Build history of the part. All positions in model axes, mm. A direction names the side the tool comes from. Give positions to 0.01 mm unless a question says otherwise; leave off trailing zeros. Order: outer loops, then holes, each group sorted by start corner. A loop starts at its lowest first (then second) coordinate and runs counter-clockwise, first axis right, second up. Notation, with made-up numbers: (70.5, -30.5) - (101.5, -30.5) arc R24 cw to (101.5, 8.5) - close; hole circle Ø6 at (-9, 7). An arc over 180 degrees is marked (long way). Use a Markdown table: item, result.
from build123d import *

# Parameters (mm, degrees)
SKETCH1_R           = 6.1
BOSS_EXTRUDE1_DEPTH = 4
BOSS_EXTRUDE2_START = 4
SKETCH1_3_R         = 20
SKETCH1_3_R_2       = 16
BOSS_EXTRUDE2_DEPTH = 12
BOSS_EXTRUDE3_DEPTH = 2
SKETCH1_5_R         = 2
BOSS_EXTRUDE4_DEPTH = 6
BOSS_EXTRUDE5_START = 4
SKETCH1_6_R         = 1.5
BOSS_EXTRUDE5_DEPTH = 10


with BuildPart() as part:
    # Sketch1 → Boss-Extrude1 (new body)
    with BuildSketch(Plane(origin=(0, 0, 0), x_dir=(1, 0, 0), z_dir=(0, 1, 0))):
        with BuildLine():
            Line((-24, 20), (-28, 20))
            Line((-28, 20), (-28, -20))
            Line((-28, -20), (-24, -20))
            ThreePointArc((-24, -20), (-21.171572875, -21.171572875), (-20, -24))
            Line((-20, -24), (-20, -28))
            Line((-20, -28), (20, -28))
            Line((20, -28), (20, -24))
            ThreePointArc((20, -24), (21.171572875, -21.171572875), (24, -20))
            Line((24, -20), (28, -20))
            Line((28, -20), (28, 20))
            Line((28, 20), (24, 20))
            ThreePointArc((24, 20), (21.171572875, 21.171572875), (20, 24))
            Line((20, 24), (20, 28))
            Line((20, 28), (-20, 28))
            Line((-20, 28), (-20, 24))
            ThreePointArc((-20, 24), (-21.171572875, 21.171572875), (-24, 20))
        make_face()
        Circle(SKETCH1_R, mode=Mode.SUBTRACT)
    extrude(amount=BOSS_EXTRUDE1_DEPTH)

    # Sketch1_3 → Boss-Extrude2 (add)
    with BuildSketch(Plane(origin=(0, 0, 0), x_dir=(1, 0, 0), z_dir=(0, 1, 0)).offset(BOSS_EXTRUDE2_START)):
        Circle(SKETCH1_3_R)
        Circle(SKETCH1_3_R_2, mode=Mode.SUBTRACT)
    extrude(amount=BOSS_EXTRUDE2_DEPTH)

    # Sketch1_4 → Boss-Extrude3 (add)
    with BuildSketch(Plane(origin=(0, 0, 0), x_dir=(1, 0, 0), z_dir=(0, 1, 0))):
        with BuildLine():
            Line((24, 30), (-24, 30))
            ThreePointArc((-24, 30), (-28.242640687, 28.242640687), (-30, 24))
            Line((-30, 24), (-30, -24))
            ThreePointArc((-30, -24), (-28.242640687, -28.242640687), (-24, -30))
            Line((-24, -30), (24, -30))
            ThreePointArc((24, -30), (28.242640687, -28.242640687), (30, -24))
            Line((30, -24), (30, 24))
            ThreePointArc((30, 24), (28.242640687, 28.242640687), (24, 30))
        make_face()
        with BuildLine():
            Line((-28, 20), (-28, 24))
            ThreePointArc((-28, 24), (-26.828427125, 26.828427125), (-24, 28))
            Line((-24, 28), (-20, 28))
            Line((-20, 28), (20, 28))
            Line((20, 28), (24, 28))
            ThreePointArc((24, 28), (26.828427125, 26.828427125), (28, 24))
            Line((28, 24), (28, 20))
            Line((28, 20), (28, -20))
            Line((28, -20), (28, -24))
            ThreePointArc((28, -24), (26.828427125, -26.828427125), (24, -28))
            Line((24, -28), (20, -28))
            Line((20, -28), (-20, -28))
            Line((-20, -28), (-24, -28))
            ThreePointArc((-24, -28), (-26.828427125, -26.828427125), (-28, -24))
            Line((-28, -24), (-28, -20))
            Line((-28, -20), (-28, 20))
        make_face(mode=Mode.SUBTRACT)
    extrude(amount=BOSS_EXTRUDE3_DEPTH)

    # Sketch1_5 → Boss-Extrude4 (add)
    with BuildSketch(Plane(origin=(0, 0, 0), x_dir=(1, 0, 0), z_dir=(0, 1, 0))):
        with BuildLine():
            Line((-24, -20), (-28, -20))
            Line((-28, -20), (-28, -24))
            ThreePointArc((-28, -24), (-26.828427125, -26.828427125), (-24, -28))
            Line((-24, -28), (-20, -28))
            Line((-20, -28), (-20, -24))
            ThreePointArc((-20, -24), (-21.171572875, -21.171572875), (-24, -20))
        make_face()
        with Locations((-24, -24)):
            Circle(SKETCH1_5_R, mode=Mode.SUBTRACT)
        with BuildLine():
            Line((20, -24), (20, -28))
            Line((20, -28), (24, -28))
            ThreePointArc((24, -28), (26.828427125, -26.828427125), (28, -24))
            Line((28, -24), (28, -20))
            Line((28, -20), (24, -20))
            ThreePointArc((24, -20), (21.171572875, -21.171572875), (20, -24))
        make_face()
        with Locations((24, -24)):
            Circle(SKETCH1_5_R, mode=Mode.SUBTRACT)
        with BuildLine():
            Line((24, 28), (20, 28))
            Line((20, 28), (20, 24))
            ThreePointArc((20, 24), (21.171572875, 21.171572875), (24, 20))
            Line((24, 20), (28, 20))
            Line((28, 20), (28, 24))
            ThreePointArc((28, 24), (26.828427125, 26.828427125), (24, 28))
        make_face()
        with Locations((24, 24)):
            Circle(SKETCH1_5_R, mode=Mode.SUBTRACT)
        with BuildLine():
            ThreePointArc((-24, 28), (-26.828427125, 26.828427125), (-28, 24))
            Line((-28, 24), (-28, 20))
            Line((-28, 20), (-24, 20))
            ThreePointArc((-24, 20), (-21.171572875, 21.171572875), (-20, 24))
            Line((-20, 24), (-20, 28))
            Line((-20, 28), (-24, 28))
        make_face()
        with Locations((-24, 24)):
            Circle(SKETCH1_5_R, mode=Mode.SUBTRACT)
    extrude(amount=BOSS_EXTRUDE4_DEPTH)

    # Sketch1_6 → Boss-Extrude5 (add)
    with BuildSketch(Plane(origin=(0, 0, 0), x_dir=(1, 0, 0), z_dir=(0, 1, 0)).offset(BOSS_EXTRUDE5_START)):
        with BuildLine():
            ThreePointArc((-2.732186624, -19.8125), (0, -25.5), (2.732186624, -19.8125))
            ThreePointArc((2.732186624, -19.8125), (0, -20), (-2.732186624, -19.8125))
        make_face()
        with Locations((0, -22)):
            Circle(SKETCH1_6_R, mode=Mode.SUBTRACT)
        with BuildLine():
            ThreePointArc((-19.8125, -2.732186624), (-20, 0), (-19.8125, 2.732186624))
            ThreePointArc((-19.8125, 2.732186624), (-25.5, 0), (-19.8125, -2.732186624))
        make_face()
        with Locations((-22, 0)):
            Circle(SKETCH1_6_R, mode=Mode.SUBTRACT)
        with BuildLine():
            ThreePointArc((-2.732186624, 19.8125), (0, 20), (2.732186624, 19.8125))
            ThreePointArc((2.732186624, 19.8125), (0, 25.5), (-2.732186624, 19.8125))
        make_face()
        with Locations((0, 22)):
            Circle(SKETCH1_6_R, mode=Mode.SUBTRACT)
        with BuildLine():
            ThreePointArc((19.8125, 2.732186624), (19.953069939, 1.369306394), (20, 0))
            ThreePointArc((20, 0), (19.953069939, -1.369306394), (19.8125, -2.732186624))
            ThreePointArc((19.8125, -2.732186624), (25.5, 0), (19.8125, 2.732186624))
        make_face()
        with Locations((22, 0)):
            Circle(SKETCH1_6_R, mode=Mode.SUBTRACT)
    extrude(amount=BOSS_EXTRUDE5_DEPTH)


solid = part.part
1) Tool access for faces 1 (the flat face through (0, 2, -29)), 2 (the flat face through (-20, 5, 26)), 3 (the flat face through (-26, 5, 20)), 4 (the flat face through (20, 5, -26)), 5 (the flat face through (-25, 6, 22)): list every direction of +Z, -Z, +X, -X, +Y, -Y with a clear straight run to the whole face (end or side of a thin tool).
Computed:
| item | result |
|---|---|
| face 1 | +Y |
| face 2 | +Z, +Y |
| face 3 | -X, +Y |
| face 4 | -Z, +Y |
| face 5 | +Z, -X, +Y |
2) Slice it at D-D (x = -17). Write the cut outline in (y, z), and give its area (3 significant figures).
Computed:
| item | result |
|---|---|
| outline | (0, -30) - (2, -30) - (2, -28) - (4, -28) - (4, -10.54) - (16, -10.54) - (16, 10.54) - (4, 10.54) - (4, 28) - (2, 28) - (2, 30) - (0, 30) - close |
| area | 485 mm² |
3) Pin check, flat tips, straight feed: P1, Ø2, axis at y = 4.5, z = -27, coming from the -X side; P2, Ø4, axis at x = -23.5, y = 10, coming from the +Z side; P3, Ø6, axis at x = -3, y = 6, coming from the +Z side. Stop position of each tip, or through.
Computed:
| item | result |
|---|---|
| P1 | stops at x = -27.46 |
| P2 | stops at z = 3.5 |
| P3 | stops at z = 28 |
4) Two-plate mould, pull along Z, no slides. Class faces 6 (the flat face through (-28, 3.5, -0.3)), 7 (the flat face through (26, 5, 20)), 8 (the cylindrical face through (-0.195, 8.93, -23.487)), 9 (the cylindrical face through (28.289, 0.986, -28.196)): +Z half, -Z half, draft (parallel to the pull), parting line (faces both ways), or undercut.
Computed:
| item | result |
|---|---|
| face 6 | draft |
| face 7 | undercut |
| face 8 | undercut |
| face 9 | -Z half |
5) Wall check: line 1 (X direction, y = 3.7, z = 24); line 2 (Z direction, x = -22, y = 8). Give the ranges that are in metal, low to high. Write a range as from..to.
Computed:
| item | result |
|---|---|
| line 1 | x = -28..-26, -22..22, 26..28 |
| line 2 | z = -3.5..-1.5, 1.5..3.5 |
6) Slice it at C-C (y = 1). Write the cut outline in (x, z).
Computed:
| item | result |
|---|---|
| outline | (-30, -24) arc R6 ccw to (-24, -30) - (24, -30) arc R6 ccw to (30, -24) - (30, 24) arc R6 ccw to (24, 30) - (-24, 30) arc R6 ccw to (-30, 24) - close; hole circle Ø4 at (-24, -24); hole circle Ø4 at (-24, 24); hole circle Ø12.2 at (0, 0); hole circle Ø4 at (24, -24); hole circle Ø4 at (24, 24) |
